from build123d import *

# Parameters (mm, degrees)
TROU_TARAUD_M3X0_51_D     = 2.5
TROU_TARAUD_M3X0_51_DEPTH = 8.5
TROU_TARAUD_M3X0_51_TIP   = 0.751075774


with BuildPart() as part:
    # Esquisse1 → Révolution1 (revolve)
    with BuildSketch(Plane.XY, mode=Mode.PRIVATE) as r_volution1_sk:
        Polygon((0, -19.5), (0, 59.5), (1.5, 59.5), (1.5, 59), (5.9, 59), (5.9, 57), (15.5, 57), (15.5, 0), (5.9, 0), (5.9, -3), (1.5, -3), (1.5, -19.5), align=None)
    revolve(r_volution1_sk.sketch.rotate(Axis((0, 0, 0), (0, 1, 0)), 90), axis=Axis((0, 0, 0), (0, 1, 0)))

    # Trou taraudé M3x0.51
    with Locations(Plane(origin=(0, 0, 0), x_dir=(-1, 0, 0), z_dir=(0, -1, 0))):
        with Locations((0, -11), (-11, 0), (0, 11), (11, 0)):
            Hole(TROU_TARAUD_M3X0_51_D / 2, depth=TROU_TARAUD_M3X0_51_DEPTH)
            with Locations((0, 0, -(TROU_TARAUD_M3X0_51_DEPTH + TROU_TARAUD_M3X0_51_TIP / 2))):  # 118° drill point
                Cone(0, TROU_TARAUD_M3X0_51_D / 2, TROU_TARAUD_M3X0_51_TIP, mode=Mode.SUBTRACT)


solid = part.part
Read the model definition and answer for the solid it produces. Units are mm, in the model's axes. A direction names the side the tool comes from. Coordinates: 2 decimals unless noted, no trailing zeros. Loops run counter-clockwise (first coordinate to the right, second up) from the corner with the lowest first, then second, coordinate; pieces in that order, holes last.
Q1. The mould has two halves that part along Z. Classify faces 4 (the face through (-0.45, 59.25, -1.43)), 5 (the face through (0, 57, 7)), 6 (the face through (-0.2, 9.12, 11.08)), 7 (the face through (-11.2, 9.12, 0.08)): +Z half, -Z half, draft (parallel to the pull), parting line (faces both ways), or undercut.
Q2. Each of these flat-tipped pins is pushed along its axis until it touches: pin 1 Ø1 at (x, z) = (-3, -10.5) entering from +Y; pin 2 Ø1 at (y, z) = (0, -3.5) entering from -X; pin 3 Ø10 at (x, z) = (12.5, -6.5) entering from -Y. Where does it stop, or does it pass through?
Q3. The part is cut by section C-C on z = -9. Write down the section's boundary in (x, y), and give its area (3 significant figures).
Q4. The part is cut by section B-B on z = 3.5. Write down the section's boundary in (x, y).
Q5. The part is cut by section D-D on x = -13. Write down the section's boundary in (y, z), and give its area (3 significant figures).
Q6. Consider probe 1 along Y at (x, z) = (2, 5.5); probe 2 along Y at (x, z) = (2, -8.5); probe 3 along Z at (x, y) = (11, 5.75). Determine where each line is inside the solid, lowest interval first.
Q7. Which of the six approach directions +Z, -Z, +X, -X, +Y, -Y give full straight-line access (tool end or side, diameter ignored) to faces 1 (the face through (-0.45, -11.37, -1.43)), 2 (the face through (-0.259, 57.986, 5.894)), 3 (the face through (0, 59.5, 0))?
Q8. The part is cut by section A-A on x = -3.5. Write down the section's boundary in (y, z), and give its area (3 significant figures).
Results below:
1. face 4: parting line
1. face 5: draft
1. face 6: undercut
1. face 7: undercut
2. pin 1: stops at y = 57
2. pin 2: stops at x = -15.21
2. pin 3: stops at y = 0
3. outline: (-12.62, 0) - (12.62, 0) - (12.62, 57) - (-12.62, 57) - close
3. area: 1,440 mm2
4. outline: (-15.1, 0) - (-4.75, 0) - (-4.75, -3) - (4.75, -3) - (4.75, 0) - (15.1, 0) - (15.1, 57) - (4.75, 57) - (4.75, 59) - (-4.75, 59) - (-4.75, 57) - (-15.1, 57) - close
5. outline: (0, -8.44) - (57, -8.44) - (57, 8.44) - (0, 8.44) - close
5. area: 962 mm2
6. probe 1: y = -3 to 59
6. probe 2: y = 0 to 57
6. probe 3: z = -10.92 to -1.25, 1.25 to 10.92
7. face 1: -Y
7. face 2: +Y
7. face 3: +Z, -Z, +X, -X, +Y
8. outline: (-3, -4.75) - (0, -4.75) - (0, -15.1) - (57, -15.1) - (57, -4.75) - (59, -4.75) - (59, 4.75) - (57, 4.75) - (57, 15.1) - (0, 15.1) - (0, 4.75) - (-3, 4.75) - close
8. area: 1,770 mm2
